Verification items for the finished model (mm, model axes). Coordinates: 2 decimals unless noted, no trailing zeros. Order: outer loops, then holes, each group sorted by start corner. A loop starts at its lowest first (then second) coordinate and runs counter-clockwise, first axis right, second up. Notation, with made-up numbers: M 60.5,11 L 101.5,11 A9 cw 101.5,16 Z; hole C -17,80.5 d6. An arc over 180 degrees is marked long. Return JSON: item names as keys, results as strings. Group by question number.
1. Section check B-B, the plane z = 35.5. Record the cut outline in (x, y), plus the area to 3 significant figures.
2. Section check C-C, the plane y = -16.5. Record the cut outline in (x, z), plus the area to 3 significant figures.
3. Section check A-A, the plane x = -37. Record the cut outline in (y, z).
4. Material ranges on line 1 along Z through (x, y) = (-33, 28); line 2 along X through (y, z) = (52, 31.25); line 3 along X through (y, z) = (-1, 35), recorded low to high.
5. Gauge pin test, flat ends, axial feed: pin 1 (5 mm diameter, centred on y = 61, z = 34.5, fed in from -X); pin 2 (4 mm diameter, centred on y = 100.5, z = 33.5, fed in from +X); pin 3 (4 mm diameter, centred on x = -31, y = -26.5, fed in from -Z). Record the tip position at first contact, or that the pin passes through.
```python
from build123d import *

# Parameters (mm, degrees)
F0_R     = 13.3568816407
F1_DEPTH = 127
F3_R     = 6.35
F4_DEPTH = 127
F6_R     = 6.5291630237
F7_DEPTH = 127


with BuildPart() as f1:
    # F0 (on Top) → F1 (new body, symmetric)
    with BuildSketch(Plane.XY):
        with Locations((-30.3778361085, 35.4953636827)):
            Circle(F0_R)
    extrude(amount=F1_DEPTH, both=True)


with BuildPart() as f4:
    # F3 (on Top) → F4 (new body, symmetric)
    with BuildSketch(Plane.XY):
        with Locations((-33.7284424831, 38.4713762078)):
            Circle(F3_R)
    extrude(amount=F4_DEPTH, both=True)


with BuildPart() as f7:
    # F6 (on Front) → F7 (new body, symmetric)
    with BuildSketch(Plane.XZ):
        with Locations((-33.6283754377, 30.9787562468)):
            Circle(F6_R)
    extrude(amount=F7_DEPTH, both=True)


solid = f7.part
```
Answers follow:
{
 "1": {"outline": "M -38.34,-127 L -28.92,-127 L -28.92,127 L -38.34,127 Z", "area": "2,390 mm^2"},
 "2": {"outline": "C -33.63,30.98 d13.06", "area": "134 mm^2"},
 "3": {"outline": "M -127,25.39 L 127,25.39 L 127,36.57 L -127,36.57 Z"},
 "4": {"line 1": "24.48 to 37.48", "line 2": "-40.15 to -27.1", "line 3": "-38.77 to -28.48"},
 "5": {"pin 1": "x = -40.08", "pin 2": "x = -27.12", "pin 3": "z = 24.48"}
}
